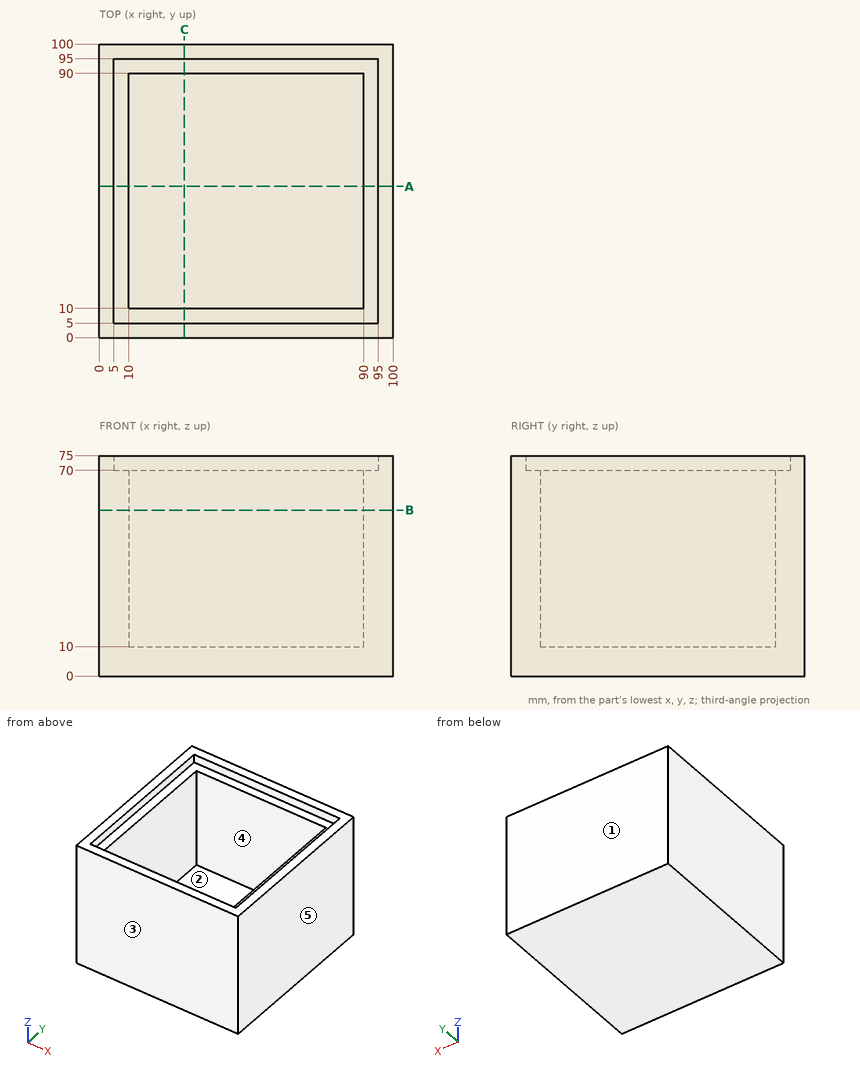
Answer from the drawing. Dimensions are ordinates in mm from the lowest x, y and z of the part. A direction names the side the tool comes from. Give positions to 0.01 mm unless a question says otherwise; leave off trailing zeros. Order: outer loops, then holes, each group sorted by start corner. A loop starts at its lowest first (then second) coordinate and runs counter-clockwise, first axis right, second up. Notation, with made-up numbers: (-6, 36.5) -> (17, 36.5) arc R22 cw to (17, 60.5) -> close; hole circle Ø7 at (46.5, 11.25). An arc over 180 degrees is marked (long way). One line per item, written item: value. Start each with the question number.
(1) For a pull along Y with two mould halves and no side action, classify the marked faces 3, 4 and 5 as released by +Y, released by -Y, zero draft, split by the parting line, or undercut.
(2) The part is cut by section A-A (y = 51.5). Determine the outline of the cut face in (x, z), and give its area (3 significant figures).
(3) A tool of negligible diameter and unlimited length cuts with its end or side. For the marked faces 1 and 2, from which of +Z, -Z, +X, -X, +Y, -Y can it reach the whole face along a straight path? Write none if from no direction.
(4) The part is cut by section B-B (z = 56.5). Determine the outline of the cut face in (x, y), and give its area (3 significant figures).
(5) Straight lines are drawn through the part: L1, parallel to Y at x = 60, z = 19; L2, parallel to Z at x = 78.5, y = 71. For each, find the intervals that lie inside material, in ascending order.
(6) Flat-ended cylindrical pins translate along their axes: P1, Ø5, axis at x = 82.5, z = 65.5, coming from the -Y side; P2, Ø1, axis at x = 32.5, y = 28, coming from the +Z side. Find the tip coordinate at first contact, or state that the pin passes through.
Taken from the geometry:
1. face 3: released by -Y
1. face 4: undercut
1. face 5: zero draft
2. outline: (0, 0) -> (100, 0) -> (100, 75) -> (95, 75) -> (95, 70) -> (90, 70) -> (90, 10) -> (10, 10) -> (10, 70) -> (5, 70) -> (5, 75) -> (0, 75) -> close
2. area: 2,250 mm^2
3. face 1: +Z, -Z, +X, -X, +Y
3. face 2: +Z
4. outline: (0, 0) -> (100, 0) -> (100, 100) -> (0, 100) -> close; hole (10, 10) -> (90, 10) -> (90, 90) -> (10, 90) -> close
4. area: 3,600 mm^2
5. L1: 0 to 10, 90 to 100
5. L2: 0 to 10
6. P1: y = 0
6. P2: z = 10
